```python
from build123d import *

# Parameters (mm, degrees)
SKETCH1_W           = 120
SKETCH1_H           = 100
BOSS_EXTRUDE1_DEPTH = 5
SKETCH2_R           = 2.5
CUT_EXTRUDE1_DEPTH  = 6
CUT_EXTRUDE3_DEPTH  = 10
BOSS_EXTRUDE3_DEPTH = 30
SKETCH8_W           = 20
SKETCH8_H           = 5
BOSS_EXTRUDE4_DEPTH = 35
SKETCH9_W           = 25
SKETCH9_H           = 10
CUT_EXTRUDE4_DEPTH  = 71
SKETCH10_W          = 35
SKETCH10_H          = 70
CUT_EXTRUDE5_DEPTH  = 120.765167123


with BuildPart() as part:
    # Sketch1 → Boss-Extrude1 (new body)
    with BuildSketch(Plane.XY):
        with Locations((60, 50)):
            Rectangle(SKETCH1_W, SKETCH1_H)
    boss_extrude1 = extrude(amount=BOSS_EXTRUDE1_DEPTH)

    # Sketch2 → Cut-Extrude1 (cut, through all)
    with BuildSketch(Plane.XY.offset(5)):
        with Locations((48.561388608, 53.909722104)):
            Circle(SKETCH2_R)
        with BuildLine():
            ThreePointArc((83.262763007, 4.351023424), (93.087143476, 12.949898455), (100.837944203, 23.456286582))
            ThreePointArc((100.837944203, 23.456286582), (96.148678733, 41.232978888), (78.371986427, 36.543713418))
            ThreePointArc((78.371986427, 36.543713418), (73.952108326, 30.552467296), (68.349775662, 25.648976576))
            ThreePointArc((68.349775662, 25.648976576), (65.157292759, 7.543506327), (83.262763007, 4.351023424))
        make_face()
    cut_extrude1 = extrude(amount=-CUT_EXTRUDE1_DEPTH, mode=Mode.SUBTRACT)

    # Sketch5 → Cut-Extrude3 (cut)
    with BuildSketch(Plane.XY.offset(5)):
        with BuildLine():
            Line((120, 70), (48.561388608, 70))
            ThreePointArc((48.561388608, 70), (39.016134462, 66.862913451), (33.192915272, 58.674915711))
            Line((33.192915272, 58.674915711), (15, 0))
            Line((15, 0), (0, 0))
            Line((0, 0), (0, 100))
            Line((0, 100), (120, 100))
            Line((120, 100), (120, 70))
        make_face()
    cut_extrude3 = extrude(amount=-CUT_EXTRUDE3_DEPTH, mode=Mode.SUBTRACT)

    # Sketch7 → Boss-Extrude3 (add)
    with BuildSketch(Plane(origin=(0, 0, 0), x_dir=(-1, 0, 0), z_dir=(0, 0, -1))):
        Polygon((-15, 0), (-32.773002065, 57.320631823), (-37.206950606, 54.737658166), (-20.234832877, 0), align=None)
        with BuildLine():
            Line((-120, 70), (-48.561388608, 70))
            ThreePointArc((-48.561388608, 70), (-46.197570118, 69.825418913), (-43.885046952, 69.305464096))
            Line((-43.885046952, 69.305464096), (-47.035737431, 64.805811769))
            ThreePointArc((-47.035737431, 64.805811769), (-47.792408669, 64.951257894), (-48.561388608, 65))
            Line((-48.561388608, 65), (-120, 65))
            Line((-120, 65), (-120, 70))
        make_face()
    boss_extrude3 = extrude(amount=BOSS_EXTRUDE3_DEPTH)

    # Sketch8 → Boss-Extrude4 (add, through all)
    with BuildSketch(Plane(origin=(0, 0, -30), x_dir=(-1, 0, 0), z_dir=(0, 0, -1))):
        with Locations((-10.234832877, 2.5)):
            Rectangle(SKETCH8_W, SKETCH8_H)
    boss_extrude4 = extrude(amount=-BOSS_EXTRUDE4_DEPTH)

    # Sketch9 → Cut-Extrude4 (cut, through all)
    with BuildSketch(Plane(origin=(0, 70, 0), x_dir=(1, 0, 0), z_dir=(0, 1, 0))):
        with Locations((102.5, 25)):
            Rectangle(SKETCH9_W, SKETCH9_H)
    cut_extrude4 = extrude(amount=-CUT_EXTRUDE4_DEPTH, mode=Mode.SUBTRACT)

    # Mirror1: Boss-Extrude1, Cut-Extrude1, Cut-Extrude3, Boss-Extrude3, Boss-Extrude4, Cut-Extrude4 across plane
    add(boss_extrude1.mirror(Plane(origin=(0, 0, 5), x_dir=(1, 0, 0), z_dir=(0, 0, -1))))
    add(cut_extrude1.mirror(Plane(origin=(0, 0, 5), x_dir=(1, 0, 0), z_dir=(0, 0, -1))), mode=Mode.SUBTRACT)
    add(cut_extrude3.mirror(Plane(origin=(0, 0, 5), x_dir=(1, 0, 0), z_dir=(0, 0, -1))), mode=Mode.SUBTRACT)
    add(boss_extrude3.mirror(Plane(origin=(0, 0, 5), x_dir=(1, 0, 0), z_dir=(0, 0, -1))))
    add(boss_extrude4.mirror(Plane(origin=(0, 0, 5), x_dir=(1, 0, 0), z_dir=(0, 0, -1))))
    add(cut_extrude4.mirror(Plane(origin=(0, 0, 5), x_dir=(1, 0, 0), z_dir=(0, 0, -1))), mode=Mode.SUBTRACT)

    # Sketch10 → Cut-Extrude5 (cut, through all)
    with BuildSketch(Plane(origin=(120, 0, 0), x_dir=(0, 0, -1), z_dir=(1, 0, 0))):
        with Locations((12.5, 35)):
            Rectangle(SKETCH10_W, SKETCH10_H)
    extrude(amount=-CUT_EXTRUDE5_DEPTH, mode=Mode.SUBTRACT)


solid = part.part
```
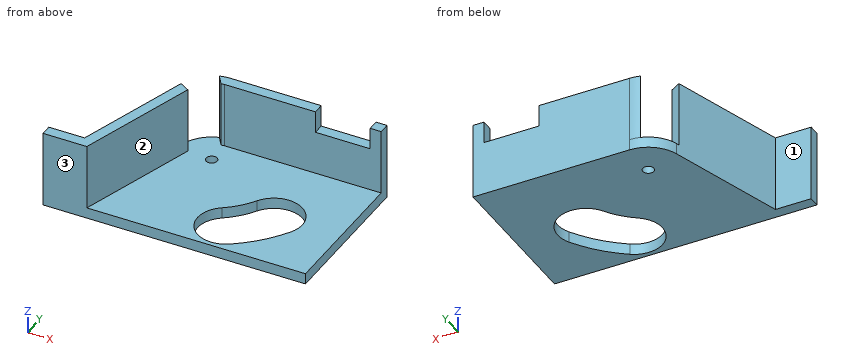
Geometry check sheet. Reference: the model listing, model coordinates, mm. Face numbers are marked on the shaded views. A direction names the side the tool comes from. Coordinates: 2 decimals unless noted, no trailing zeros. Order: outer loops, then holes, each group sorted by start corner. A loop starts at its lowest first (then second) coordinate and runs counter-clockwise, first axis right, second up. Notation, with made-up numbers: (-11.5, -1) - (43.5, -1) arc R31 cw to (43.5, 29) - close; hole circle Ø8 at (26, 66). An arc over 180 degrees is marked (long way). Answer in a Markdown table with one row per item. Add a question column.
1. Section check C-C (x = 88). Enter the section's corners in (y, z), plus the area to 3 significant figures.
2. Section check B-B (y = 30). Enter the section's corners in (x, z).
3. Gauge pin test, flat ends, axial feed: pin 1 Ø8 at (y, z) = (47, 36.5) entering from +X; pin 2 Ø12 at (x, y) = (41, 35.5) entering from +Z; pin 3 Ø2.5 at (x, y) = (96.5, 67.5) entering from +Z. Record the tip position at first contact, or that the pin passes through.
4. Section check A-A (z = 19.5). Enter the section's corners in (x, y).
5. Access from +Z, -Z, +X, -X, +Y, -Y to the whole of each face (thin tool, end or side, straight path). Record for the marked faces 1, 2 and 3.
6. Material ranges on L1, parallel to Z at x = 112, y = 36.5; L2, parallel to Y at x = 63, z = 34.5; L3, parallel to Y at x = 12, z = 10, recorded low to high. Write a range as [from, to].
7. Section check D-D (z = 37). Enter the section's corners in (x, y), plus the area to 3 significant figures.
Data:
| question | item | result |
|---|---|---|
| 1 | outline | (0, 5) - (8.03, 5) - (8.03, 10) - (0, 10) - close; (42.9, 5) - (70, 5) - (70, 40) - (65, 40) - (65, 10) - (42.9, 10) - close |
| 1 | area | 326 mm² |
| 2 | outline | (24.3, 5) - (73.43, 5) - (73.43, 10) - (29.54, 10) - (29.54, 40) - (24.3, 40) - close; (102.6, 5) - (120, 5) - (120, 10) - (102.6, 10) - close |
| 3 | pin 1 | stops at x = 36.05 |
| 3 | pin 2 | stops at z = 10 |
| 3 | pin 3 | stops at z = 30 |
| 4 | outline | (0.23, 0) - (20.23, 0) - (37.21, 54.74) - (32.77, 57.32) - (16.55, 5) - (0.23, 5) - close; (43.89, 69.31) - (47.04, 64.81) arc R6.09 cw to (48.56, 65) - (120, 65) - (120, 70) - (48.56, 70) arc R16.09 ccw to start |
| 5 | face 1 | +Z, -Z, -X, +Y |
| 5 | face 2 | +Z, +X, -Y |
| 5 | face 3 | +Z, -Z, +X, -X, -Y |
| 6 | L1 | z = [5, 10] |
| 6 | L2 | y = [65, 70] |
| 6 | L3 | y = [0, 5] |
| 7 | outline | (0.23, 0) - (20.23, 0) - (37.21, 54.74) - (32.77, 57.32) - (16.55, 5) - (0.23, 5) - close; (43.89, 69.31) - (47.04, 64.81) arc R6.09 cw to (48.56, 65) - (90, 65) - (90, 70) - (48.56, 70) arc R16.09 ccw to start; (115, 65) - (120, 65) - (120, 70) - (115, 70) - close |
| 7 | area | 619 mm² |
